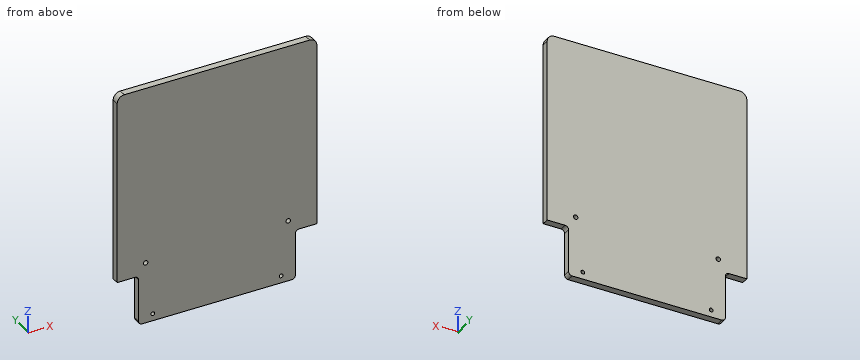
from build123d import *

# Parameters (mm, degrees)
SKETCH1_W                      = 355.6
SKETCH1_H                      = 428.625
BOSS_EXTRUDE1_DEPTH            = 12.7
FILLET1_R                      = 12.7
SKETCH3_W                      = 38.1
SKETCH3_H                      = 88.9
CUT_EXTRUDE2_DEPTH             = 558.074537764
FILLET2_R                      = 6.35
H_0_266_DIAMETER_HOLE1_D       = 6.7564
F_5_16_0_3125_DIAMETER_HOLE1_D = 7.9375


with BuildPart() as part:
    # Sketch1 → Boss-Extrude1 (new body)
    with BuildSketch(Plane(origin=(0, 0, 0), x_dir=(1, 0, 0), z_dir=(0, 1, 0))):
        with Locations((177.8, 214.3125)):
            Rectangle(SKETCH1_W, SKETCH1_H)
    extrude(amount=BOSS_EXTRUDE1_DEPTH)

    # Fillet1
    fillet1_edges = [part.edges().sort_by_distance(p)[0] for p in [
        (355.6, 6.35, 0),
        (0, 6.35, 0),
    ]]
    fillet(fillet1_edges, radius=FILLET1_R)

    # Sketch3 → Cut-Extrude2 (cut, through all)
    with BuildSketch(Plane(origin=(0, 12.7, 0), x_dir=(1, 0, 0), z_dir=(0, 1, 0))):
        with Locations((19.05, 384.175)):
            Rectangle(SKETCH3_W, SKETCH3_H)
        with Locations((336.55, 384.175)):
            Rectangle(SKETCH3_W, SKETCH3_H)
    extrude(amount=-CUT_EXTRUDE2_DEPTH, mode=Mode.SUBTRACT)

    # Fillet2
    fillet2_edges = [part.edges().sort_by_distance(p)[0] for p in [
        (38.1, 6.35, -428.625),
        (38.1, 6.35, -339.725),
        (317.5, 6.35, -428.625),
        (317.5, 6.35, -339.725),
    ]]
    fillet(fillet2_edges, radius=FILLET2_R)

    # H (0.266) Diameter Hole1 (through all)
    with Locations(Plane(origin=(0, 12.7, 0), x_dir=(1, 0, 0), z_dir=(0, 1, 0))):
        with Locations((63.5, 415.925), (292.1, 415.925)):
            Hole(H_0_266_DIAMETER_HOLE1_D / 2)

    # 5/16 (0.3125) Diameter Hole1 (through all)
    with Locations(Plane(origin=(0, 0, 0), x_dir=(-1, 0, 0), z_dir=(0, -1, 0))):
        with Locations((-50.8, 319.0875), (-304.8, 319.0875)):
            Hole(F_5_16_0_3125_DIAMETER_HOLE1_D / 2)


solid = part.part
Read the model definition and answer for the solid it produces. Units are mm, in the model's axes. Coordinates: 2 decimals unless noted, no trailing zeros. Write item = value, one per line. Start each with the question number.
1) Given P1, Ø4, axis at y = 4.5, z = -372.5, coming from the -X side, flat-ended and moving along its own axis, determine where the tip first touches the part or whether it passes through.
2) Find the intervals of material crossed by L1, parallel to Z at x = 292.1, y = 4 (3 decimals); L2, parallel to Z at x = 50.8, y = 10.25 (3 decimals); L3, parallel to X at y = 12, z = -408, in increasing order. Write a range as from..to.
3) The part is cut by section A-A, the plane y = 8.25. State how many separate pieces and enclosed holes the cut face has, plus the area to 3 significant figures.
Result:
q1.P1 = 38.1
q2.L1 = -428.625..-419.303, -412.547..0
q2.L2 = -428.625..-323.056, -315.119..0
q2.L3 = 38.1..317.5
q3.separate_pieces = 1
q3.enclosed_holes = 4
q3.area = 145,000 mm²
